```python
from build123d import *

# Parameters (mm, degrees)
SKETCH1_R        = 10
SMALLRING_DEPTH  = 12
SKETCH4_R        = 19
SKETCH4_R_2      = 2
BIGRING_DEPTH    = 5
SKETCH42_R       = 3.8125
SHAFT_HOLE_DEPTH = 17
SKETCH43_W       = 3
SKETCH43_H       = 4
KEYWAY_DEPTH     = 17


with BuildPart() as part:
    # Sketch1 → SmallRing (new body)
    with BuildSketch(Plane(origin=(0, 0, 0), x_dir=(0, 0, -1), z_dir=(1, 0, 0))):
        Circle(SKETCH1_R)
    extrude(amount=SMALLRING_DEPTH)

    # Sketch4 → BigRing (add)
    with BuildSketch(Plane.ZY):
        Circle(SKETCH4_R)
        with Locations((-10.606601718, 10.606601718)):
            Circle(SKETCH4_R_2, mode=Mode.SUBTRACT)
        with Locations((10.606601718, 10.606601718)):
            Circle(SKETCH4_R_2, mode=Mode.SUBTRACT)
        with Locations((10.606601718, -10.606601718)):
            Circle(SKETCH4_R_2, mode=Mode.SUBTRACT)
        with Locations((-10.606601718, -10.606601718)):
            Circle(SKETCH4_R_2, mode=Mode.SUBTRACT)
    extrude(amount=BIGRING_DEPTH)

    # Sketch42 → Shaft Hole (cut)
    with BuildSketch(Plane(origin=(12, 0, 0), x_dir=(0, 0, -1), z_dir=(1, 0, 0))):
        Circle(SKETCH42_R)
    extrude(amount=-SHAFT_HOLE_DEPTH, mode=Mode.SUBTRACT)

    # Sketch43 → KeyWay (cut)
    with BuildSketch(Plane(origin=(12, 0, 0), x_dir=(0, 0, -1), z_dir=(1, 0, 0))):
        with Locations((0, 3.8125)):
            Rectangle(SKETCH43_W, SKETCH43_H)
    extrude(amount=-KEYWAY_DEPTH, mode=Mode.SUBTRACT)


solid = part.part
```
The listing builds one solid part. Answer for the finished solid, in the listing's coordinates (mm). A direction names the side the tool comes from. Coordinates: 2 decimals unless noted, no trailing zeros. Loops run counter-clockwise (first coordinate to the right, second up) from the corner with the lowest first, then second, coordinate; pieces in that order, holes last. Notation, with made-up numbers: (67.25, 1) - (72.25, 1) arc R18 ccw to (72.25, 29) - close; hole circle Ø4 at (-11, 29). An arc over 180 degrees is marked (long way). Use a Markdown table: item, result. Add a question column.
1) The mould has two halves that part along Y. Classify faces 1 (the cylindrical face through (-2.5, 9.4, -12.2)), 2 (the cylindrical face through (-2.465, -16.856, 8.767)), 3 (the flat face through (0, -8, 8)): released by +Y, released by -Y, zero draft, split by the parting line, or undercut.
2) The part is cut by section A-A, the plane y = 0. Give the vertices of the cut face in (x, z), and give its area (3 significant figures).
3) Find the intervals of material crossed by line 1 (Y direction, x = 6, z = 0); line 2 (X direction, y = 12, z = 4); line 3 (Z direction, x = 3.75, y = 2.5), in increasing order.
4) The part is cut by section B-B, the plane z = 0. Give the vertices of the cut face in (x, y).
5) For faces 4 (the flat face through (4, 5, 1.5)), 5 (the cylindrical face through (5.92, -9.76, 2.17)), 6 (the flat face through (-5, -4, 0)), determine the directions among +Z, -Z, +X, -X, +Y, -Y from which every point of the face is accessible in a straight line to the end or side of a thin tool.
6) The part is cut by section C-C, the plane x = 10.75. Give the vertices of the cut face in (y, z) (1 decimal).
7) The part is cut by section D-D, the plane z = 11. Give the vertices of the cut face in (x, y), and give its area (3 significant figures).
8) Given pin 1 (6.5 mm diameter, centred on y = 10.61, z = 10.61, fed in from +X); pin 2 (1.5 mm diameter, centred on x = 0.5, y = -7, fed in from -Z); pin 3 (10 mm diameter, centred on x = 10, y = -5.5, fed in from +Z), each flat-ended and moving along its own axis, determine where each tip first touches the part or whether it passes through.
Here are the results:
| question | item | result |
|---|---|---|
| 1 | face 1 | undercut |
| 1 | face 2 | split by the parting line |
| 1 | face 3 | zero draft |
| 2 | outline | (-5, -19) - (0, -19) - (0, -10) - (12, -10) - (12, -3.81) - (-5, -3.81) - close; (-5, 3.81) - (12, 3.81) - (12, 10) - (0, 10) - (0, 19) - (-5, 19) - close |
| 2 | area | 300 mm^2 |
| 3 | line 1 | y = -10 to -3.81, 5.81 to 10 |
| 3 | line 2 | x = -5 to 0 |
| 3 | line 3 | z = -9.68 to -2.88, 2.88 to 9.68 |
| 4 | outline | (-5, -19) - (0, -19) - (0, -10) - (12, -10) - (12, -3.81) - (-5, -3.81) - close; (-5, 5.81) - (12, 5.81) - (12, 10) - (0, 10) - (0, 19) - (-5, 19) - close |
| 5 | face 4 | +X, -X |
| 5 | face 5 | +X |
| 5 | face 6 | +Z, -Z, -X, +Y, -Y |
| 6 | outline | circle Ø20 at (0, 0); hole (3.5, -1.5) - (5.8, -1.5) - (5.8, 1.5) - (3.5, 1.5) arc R3.8 ccw (long way) to start |
| 7 | outline | (-5, -15.49) - (0, -15.49) - (0, -12.57) - (-5, -12.57) - close; (-5, -8.65) - (0, -8.65) - (0, 8.65) - (-5, 8.65) - close; (-5, 12.57) - (0, 12.57) - (0, 15.49) - (-5, 15.49) - close |
| 7 | area | 116 mm^2 |
| 8 | pin 1 | stops at x = 0 |
| 8 | pin 2 | stops at z = -17.87 |
| 8 | pin 3 | stops at z = 9.99 |
